Geometry check sheet. Reference: drawing and pictorial views, mm from the part's lowest x, y, z. A direction names the side the tool comes from. Give positions to 0.01 mm unless a question says otherwise; leave off trailing zeros. Write each loop counter-clockwise with the first axis right and the second up, starting at its lowest first coordinate (ties: lowest second). Pieces come first, ordered by that corner, then holes.
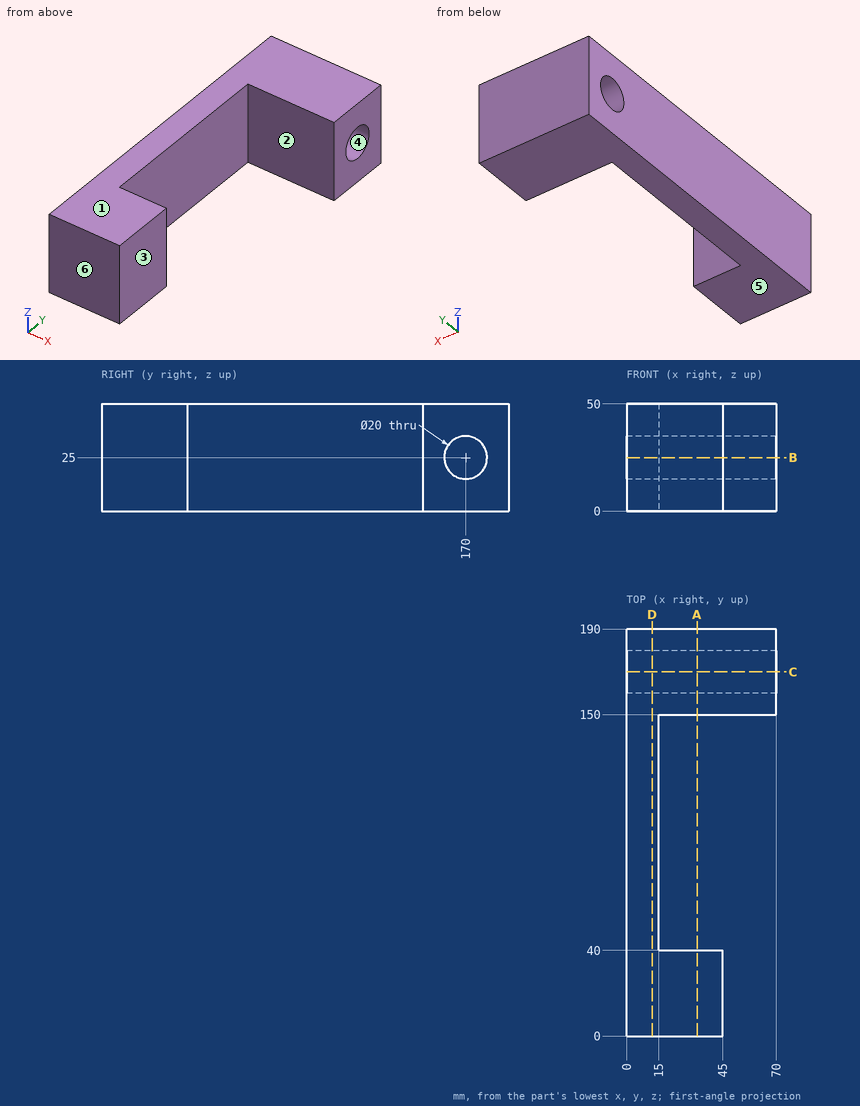
Item 1: Scan lines: line 1 along Y through (x, z) = (50.5, 25); line 2 along Y through (x, z) = (43, 33); line 3 along Y through (x, z) = (26, 48). Record each from-to range of solid material in increasing order.
Answer key:
line 1: y = 150 to 160, 180 to 190
line 2: y = 0 to 40, 150 to 164, 176 to 190
line 3: y = 0 to 40, 150 to 190
Item 2: Sectioned sample at A-A on x = 33. Record the cut outline in (y, z).
Answer key:
outline: (0, 0) - (40, 0) - (40, 50) - (0, 50) - close; (150, 0) - (190, 0) - (190, 50) - (150, 50) - close; hole circle Ø20 at (170, 25)
Item 3: Sectioned sample at C-C on y = 170. Record the cut outline in (x, z), then the cut area to 3 significant figures.
Answer key:
outline: (0, 0) - (70, 0) - (70, 15) - (0, 15) - close; (0, 35) - (70, 35) - (70, 50) - (0, 50) - close
area: 2,100 mm2
Item 4: Release check for a two-part mould opening along Z. For the marked faces 4, 5 and 6 record: released by +Z, released by -Z, zero draft, split by the parting line, or undercut.
Answer key:
face 4: undercut
face 5: released by -Z
face 6: zero draft
Item 5: Set-up check for the marked faces 1, 2 and 3: record each of +Z, -Z, +X, -X, +Y, -Y from which the full face is reachable in a straight line by a thin tool's end or side.
Answer key:
face 1: +Z, +X, -X, +Y, -Y
face 2: +Z, -Z, +X
face 3: +Z, -Z, +X, -Y
Item 6: Depth check by flat-ended pin: pin 1 (12 mm diameter, centred on y = 34.5, z = 12, fed in from +X); pin 2 (3 mm diameter, centred on y = 79, z = 33.5, fed in from +X). Enter the tip coordinate at first touch or a pass-through.
Answer key:
pin 1: stops at x = 45
pin 2: stops at x = 15
Item 7: Sectioned sample at B-B on z = 25. Record the cut outline in (x, y), then the cut area to 3 significant figures.
Answer key:
outline: (0, 0) - (45, 0) - (45, 40) - (15, 40) - (15, 150) - (70, 150) - (70, 160) - (0, 160) - close; (0, 180) - (70, 180) - (70, 190) - (0, 190) - close
area: 4,850 mm2
Item 8: Sectioned sample at D-D on x = 12. Record the cut outline in (y, z), then the cut area to 3 significant figures.
Answer key:
outline: (0, 0) - (190, 0) - (190, 50) - (0, 50) - close; hole circle Ø20 at (170, 25)
area: 9,190 mm2
